Drawing for the job (mm, zero at the part's lowest x, y, z). Coordinates: 2 decimals unless noted, no trailing zeros. Order: outer loops, then holes, each group sorted by start corner. A loop starts at its lowest first (then second) coordinate and runs counter-clockwise, first axis right, second up.
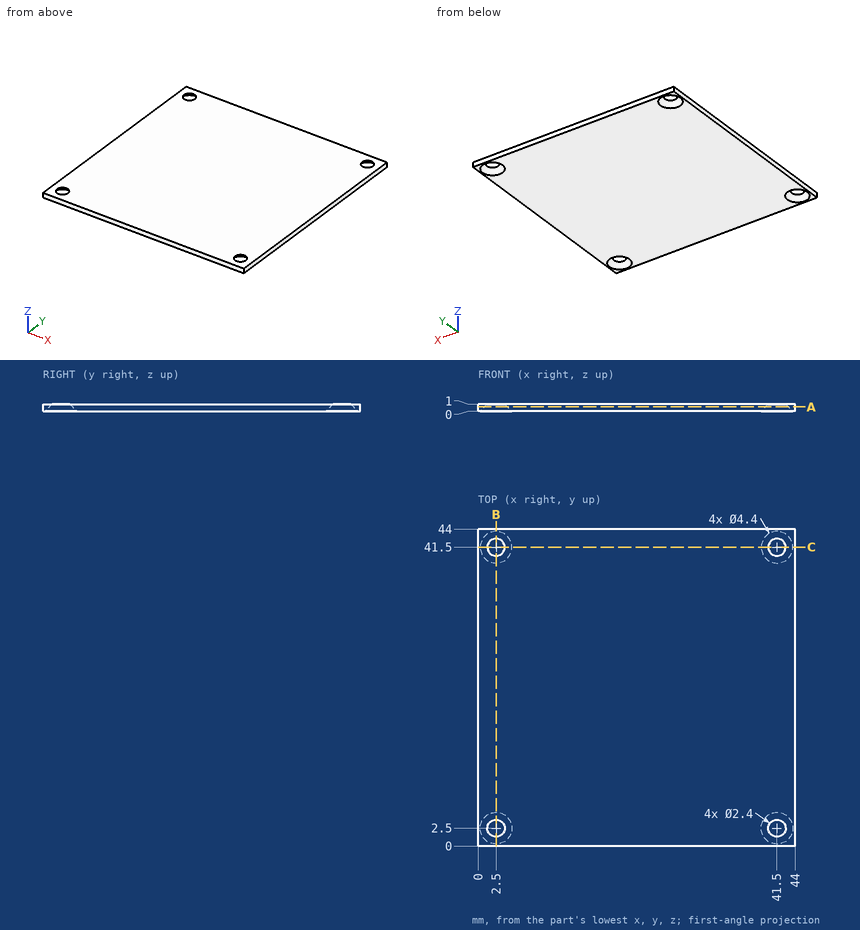
1) Slice it at A-A (z = 0.6). List the corners of the cut face in (x, y), plus the area to 3 significant figures.
2) Slice it at B-B (x = 2.5). List the corners of the cut face in (y, z).
3) Drill centre lines: probe 1 along X at (y, z) = (3, 0.25); probe 2 along X at (y, z) = (3.5, 0.5); probe 3 along Y at (x, z) = (3, 0.5). Where is each one in solid material? Low to high.
Worked out:
1. outline: (0, 0) - (44, 0) - (44, 44) - (0, 44) - close; hole circle Ø3.2 at (2.5, 2.5); hole circle Ø3.2 at (2.5, 41.5); hole circle Ø3.2 at (41.5, 2.5); hole circle Ø3.2 at (41.5, 41.5)
1. area: 1,900 mm2
2. outline: (0, 0) - (0.3, 0) - (1.3, 1) - (0, 1) - close; (3.7, 1) - (4.7, 0) - (39.3, 0) - (40.3, 1) - close; (42.7, 1) - (43.7, 0) - (44, 0) - (44, 1) - close
3. probe 1: x = 0 to 0.62, 4.38 to 39.62, 43.38 to 44
3. probe 2: x = 0 to 1.13, 3.87 to 40.13, 42.87 to 44
3. probe 3: y = 0 to 0.88, 4.12 to 39.88, 43.12 to 44
